For this review, take the finished solid that the model builds, in its own axes (mm). A direction names the side the tool comes from. Coordinates: 2 decimals unless noted, no trailing zeros. Write each loop counter-clockwise with the first axis right and the second up, starting at its lowest first coordinate (ties: lowest second). Pieces come first, ordered by that corner, then holes. Notation, with made-up numbers: M 28,3.5 L 32,3.5 A15 cw 32,18.5 Z; hole C -15,-25.5 d9. An arc over 180 degrees is marked long. One line per question, with ' | ' between items.
from build123d import *

# Parameters (mm, degrees)
F0_W     = 660.4
F0_H     = 50.8
F1_DEPTH = 19.05
F2_DEPTH = 19.05
F0_H_2   = 742.95
F3_DEPTH = 19.05


with BuildPart() as f1:
    # F0 (on Right) → F1 (new body)
    with BuildSketch(Plane.YZ):
        with Locations((24.521003, 353.902827)):
            Rectangle(F0_W, F0_H)
    extrude(amount=F1_DEPTH)



with BuildPart() as f2:
    # F0 (on Right) → F2 (new body)
    with BuildSketch(Plane.YZ):
        with Locations((24.521003, 353.902827)):
            Rectangle(F0_W, F0_H)
    extrude(amount=-F2_DEPTH)


with BuildPart() as f1_1:
    add(f1.part)

    add(f2.part)  # F3 merges F2
    # F0 (on Right) → F3 (join)
    with BuildSketch(Plane.YZ):
        with Locations((24.521003, 353.902827)):
            Rectangle(F0_W, F0_H)
        with Locations((24.521003, -42.972173)):
            Rectangle(F0_W, F0_H_2)
    extrude(amount=F3_DEPTH)


solid = f1_1.part
1) We need section A-A on y = -197. State the section outline as (x, z) points, then the cut area to 3 significant figures.
Responses:
outline: M -19.05,328.5 L 0,328.5 L 0,-414.45 L 19.05,-414.45 L 19.05,379.3 L -19.05,379.3 Z | area: 16,100 mm^2
2) Machinability: for faces 1 (the flat face through (0, 20, -38)), 2 (the flat face through (19.05, 20, -12)), which of the approach directions +Z, -Z, +X, -X, +Y, -Y give a long, thin tool a straight path to every point of the face, cutting with its end or side? Answer none if there is none.
Responses:
face 1: -Z, -X, +Y, -Y | face 2: +Z, -Z, +X, +Y, -Y
3) Insertion check: pin 1 Ø9.5 at (x, y) = (-14, -86) entering from -Z; pin 2 Ø6 at (x, z) = (-2, -182.5) entering from -Y; pin 3 Ø1 at (y, z) = (272.5, -56.5) entering from -X. Each pin has a flat end and moves straight along its axis. Give the tip position at first contact, or say it passes through.
Responses:
pin 1: z = 328.5 | pin 2: y = -305.68 | pin 3: x = 0
4) We need section B-B on z = -138.5. State the section outline as (x, y) points, then the cut area to 3 significant figures.
Responses:
outline: M 0,-305.68 L 19.05,-305.68 L 19.05,354.72 L 0,354.72 Z | area: 12,600 mm^2
5) To check wall thickness, follow line 1 along X through (y, z) = (-261, -220); line 2 along Z through (x, y) = (-11.5, -226.5). State the ranges of each line that lie inside material, in increasing order. Write a range as [from, to].
Responses:
line 1: [0, 19.05] | line 2: [328.5, 379.3]
